Could you check a few things on this model? Use its own coordinates, in mm. Face numbers are marked on the shaded views. A direction names the side the tool comes from. Give positions to 0.01 mm unless a question says otherwise; leave off trailing zeros. Write each loop counter-clockwise with the first axis right and the second up, starting at its lowest first coordinate (ties: lowest second). Pieces come first, ordered by that corner, then holes. Notation, with made-up numbers: (86, 69) - (138, 69) arc R32 cw to (138, 106) - close; hole circle Ø7 at (80.5, 33.25). An arc over 180 degrees is marked (long way). Use one line per item in the form item = value.
Autodesk Inventor part; units mm, degrees
ref_plane "YZ Plane" through (0, 0, 0) normal (1, 0, 0) x (0, 1, 0)
ref_plane "XZ Plane" through (0, 0, 0) normal (0, 1, 0) x (-1, 0, 0)
ref_plane "XY Plane" through (0, 0, 0) normal (0, 0, 1) x (1, 0, 0)
sketch "Sketch1" plane through (0, 0, 0) normal (1, 0, 0) x (0, 1, 0)
  line L0 (0, 0) -> (0, -9.25)
  line L1 (0, 0) -> (0, 9.25)
  line L2 (0, -9.25) -> (14.25, -9.25)
  line L3 (14.25, -9.25) -> (14.25, -4.75)
  line L4 (14.25, -4.75) -> (0, 9.25)
  dimension "d0" = 9.25
  dimension "d1" = 9.25
  dimension "d2" = 14.25
  dimension "d3" = 4.5
sketch "Sketch2" plane through (0, 0, 0) normal (0, 0, 1) x (1, 0, 0)
  line L0 (0, 0) -> (14.125, 0) construction
  line L1 (0, 0) -> (-14.125, 0) construction
  line L2 (-14.125, 0) -> (-9.625, 0)
  line L3 (14.125, 0) -> (9.625, 0)
  arc A0 (14.125, 0) -> (-14.125, 0) centre (0, 0) ccw
  line L4 (0, 0) -> (0, 5) construction
  line L5 (-9.625, 0) -> (0, 5)
  line L6 (0, 5) -> (9.625, 0)
  line L7 (-25, 30) -> (25, 30)
  line L8 (25, 30) -> (25, -20)
  line L9 (25, -20) -> (-25, -20)
  line L10 (-25, -20) -> (-25, 30)
  line L11 (-25, 30) -> (25, -20) construction
  line L12 (25, 30) -> (-25, -20) construction
  dimension "d6" = 4.5
  dimension "d7" = 4.5
  dimension "d8" = 14.125
  dimension "d9" = 5
  dimension "d12" = 50
  dimension "d13" = 50
extrude "Extrusion1" add sketch "Sketch1" along normal mid plane 28.25
extrude "Extrusion2" cut sketch "Sketch2" along normal mid plane 28.25
equation "\"d1\" = d0"
equation "\"d10\" = 2 * d8"
equation "\"d14\" = 2 * d8"
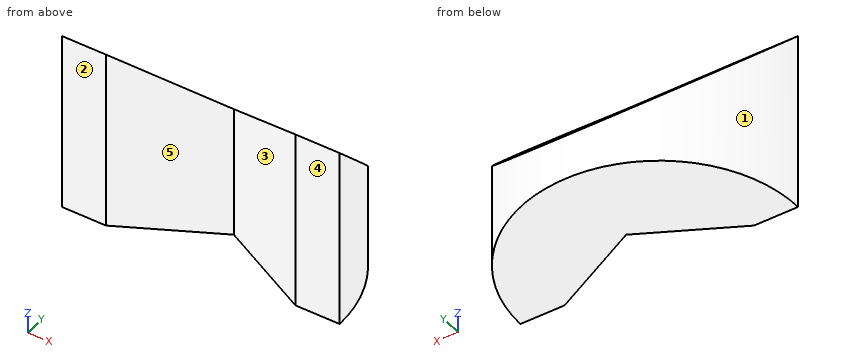
1. Imagine slicing it at D-D, the plane z = -2.75. List the corners of the cut face in (x, y) for me (3 decimals).
Response values:
outline = (-14.125, 0) - (-9.625, 0) - (0, 5) - (9.625, 0) - (14.125, 0) arc R14.125 ccw to (7.094, 12.214) - (-7.094, 12.214) arc R14.125 ccw to start
2. Imagine slicing it at B-B, the plane z = -8. List the corners of the cut face in (x, y) for me (3 decimals), and give its area (3 significant figures).
Response values:
outline = (-14.125, 0) - (-9.625, 0) - (0, 5) - (9.625, 0) - (14.125, 0) arc R14.125 ccw to start
area = 265 mm²
3. If I drill on line 1 (X direction, y = 3.5, z = 0.5); line 2 (Z direction, x = 2, y = 13.75); line 3 (Z direction, x = 6.25, y = 2.5), over which ranges is the centre line in solid material (lowest first)? Write a range as from..to.
Response values:
line_1 = -13.68..-2.89, 2.89..13.68
line_2 = -9.25..-4.26
line_3 = -9.25..6.79
4. Which directions (+Z, -Z, +X, -X, +Y, -Y) give clear straight access to the entire face, cutting with the end or side of a thin tool? Please do the marked faces 4 and 5.
Response values:
face_4 = +Z, -Z, +X, -X, -Y
face_5 = +Z, -Z, -Y
5. For pin 1 (1 mm diameter, centred on x = 7.5, y = 5.5, fed in from +Z); pin 2 (1.5 mm diameter, centred on y = 4, z = 6, fed in from -X); pin 3 (10 mm diameter, centred on x = 4, z = 4, fed in from +Y); pin 4 (8 mm diameter, centred on x = -11, y = 1.5, fed in from +Z), each with a flat end and sliding along its axis, tell me the tip position at first contact or that it passes through.
Response values:
pin_1 = 4.34
pin_2 = -13.75
pin_3 = 10.43
pin_4 = 9.25
6. Imagine slicing it at C-C, the plane x = -1.5. List the corners of the cut face in (y, z) for me, and give its area (3 significant figures).
Response values:
outline = (4.22, -9.25) - (14.05, -9.25) - (14.05, -4.55) - (4.22, 5.1) - close
area = 93.6 mm²
7. If we mould it in two halves opening along X, with no side actions, what happens to the marked faces 1, 2 and 3? For each: pulls with the +X half, pulls with the -X half, needs draft (parallel to the pull), parting line crosses it, or undercut.
Response values:
face_1 = parting line crosses it
face_2 = needs draft
face_3 = undercut
8. Imagine slicing it at A-A, the plane y = 2.25. List the corners of the cut face in (x, z) for me.
Response values:
outline = (-13.94, -9.25) - (-5.29, -9.25) - (-5.29, 7.04) - (-13.94, 7.04) - close; (5.29, -9.25) - (13.94, -9.25) - (13.94, 7.04) - (5.29, 7.04) - close
